For this review, take the finished solid that the model builds, in its own axes (mm). Face numbers are marked on the shaded views. A direction names the side the tool comes from. Coordinates: 2 decimals unless noted, no trailing zeros. Loops run counter-clockwise (first coordinate to the right, second up) from the corner with the lowest first, then second, coordinate; pieces in that order, holes last. Notation, with made-up numbers: M -30,0.25 L 29,0.25 A7 cw 29,13.25 Z; hole C 3.25,84 d3. An arc over 180 degrees is marked long. Answer as a JSON object with one key per item and string values. Group by question number.
Item 1: Wall thickness on L1, parallel to X at y = 32.5, z = 8.5; L2, parallel to X at y = 25.5, z = 23.5; L3, parallel to Y at x = 141.15, z = 5.75 (3 decimals): over which ranges is each line inside the solid? List them lowest first. Write a range as from..to.
Item 2: Add section A-A (y = 26.35). State the section outline as (x, z) points.
Item 3: Add section C-C (x = 49). State the section outline as (y, z) points (3 decimals).
Item 4: Tool access review of the marked faces 4, 5 and 6: name each direction out of +Z, -Z, +X, -X, +Y, -Y from which nothing blocks a thin tool from reaching the whole face with its end or side.
Item 5: Mouldability with a two-part tool opening along X and no side actions: class the marked faces 1, 2 and 3 as +X half, -X half, draft (parallel to the pull), parting line (faces both ways), or undercut.
Item 6: Insertion check: pin 1 (4 mm diameter, centred on x = 108.5, y = 29.5, fed in from +Z); pin 2 (6.5 mm diameter, centred on x = 61.5, y = 3.5, fed in from -Z); pin 3 (1.7 mm diameter, centred on x = 67.5, y = 1.5, fed in from +Z). Each pin has a flat end and moves straight along its axis. Give the tip position at first contact, or say it passes through.
Item 7: Add section D-D (x = 13.85). Count the separate pieces of the cut face and the enclosed holes in it, then the cut area to 3 significant figures.
Item 8: Add section B-B (z = -14). State the section outline as (x, y) points.
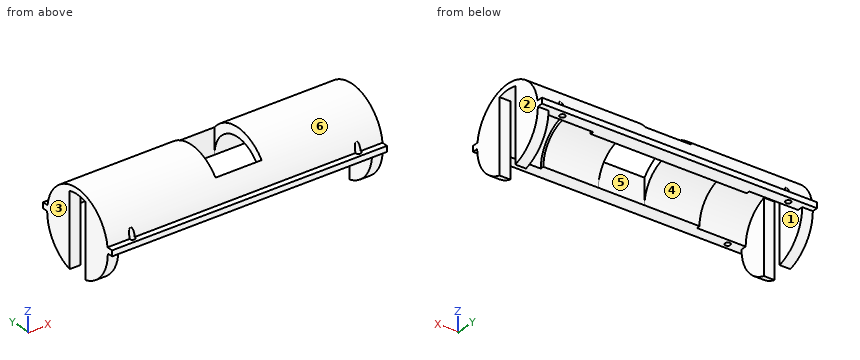
from build123d import *

# Parameters (mm, degrees)
BOSS_EXTRUDE1_DEPTH     = 155
CUT_EXTRUDE1_DEPTH      = 33.5
CUT_EXTRUDE2_START      = -33.5
CUT_EXTRUDE2_DEPTH      = 33.5
CUT_EXTRUDE3_DEPTH      = 166.346214426
CUT_EXTRUDE3_DEPTH_BACK = 166.346214426
SKETCH4_W               = 26
SKETCH4_H               = 36
CUT_EXTRUDE4_DEPTH      = 166.346214426
CUT_EXTRUDE4_DEPTH_BACK = 166.346214426
SKETCH5_R               = 1.5
BOSS_EXTRUDE2_START     = -6
BOSS_EXTRUDE2_DEPTH     = 6


with BuildPart() as part:
    # Sketch1 → Boss-Extrude1 (new body)
    with BuildSketch(Plane(origin=(0, 0, 0), x_dir=(0, 0, -1), z_dir=(1, 0, 0))):
        with BuildLine():
            Line((-6.678129735, 49.283191466), (-6.514064867, 52.7))
            Line((-6.514064867, 52.7), (-3.339064867, 52.7))
            Line((-3.339064867, 52.7), (-3.339064867, 44.35))
            ThreePointArc((-3.339064867, 44.35), (-21.339064867, 26.35), (-3.339064867, 8.35))
            Line((-3.339064867, 8.35), (-3.339064867, 0))
            Line((-3.339064867, 0), (-6.514064867, 0))
            Line((-6.514064867, 0), (-6.514064867, 3.393519434))
            ThreePointArc((-6.514064867, 3.393519434), (-26.513916757, 26.267145213), (-6.678129735, 49.283191466))
        make_face()
    extrude(amount=BOSS_EXTRUDE1_DEPTH)

    # Sketch2 → Cut-Extrude1 (cut)
    with BuildSketch(Plane(origin=(155, 0, 0), x_dir=(0, 0, -1), z_dir=(1, 0, 0))):
        with BuildLine():
            Line((-3.339064867, 46.35), (-3.339064867, 6.35))
            ThreePointArc((-3.339064867, 6.35), (-23.339064867, 26.35), (-3.339064867, 46.35))
        make_face()
    extrude(amount=-CUT_EXTRUDE1_DEPTH, mode=Mode.SUBTRACT)

    # Sketch3 → Cut-Extrude2 (cut)
    with BuildSketch(Plane.ZY.offset(CUT_EXTRUDE2_START)):
        with BuildLine():
            Line((3.339064867, 46.35), (3.339064867, 6.35))
            ThreePointArc((3.339064867, 6.35), (23.339064867, 26.35), (3.339064867, 46.35))
        make_face()
    extrude(amount=CUT_EXTRUDE2_DEPTH, mode=Mode.SUBTRACT)

    # Sketch4 → Cut-Extrude3 (cut, two sides: drawn at the far end of the back side and taken through both)
    with BuildSketch(Plane(origin=(0, 0, 3.339064867), x_dir=(-1, 0, 0), z_dir=(0, 0, -1)).offset(-CUT_EXTRUDE3_DEPTH_BACK)):
        with Locations((-77.5, 26.35)):
            Rectangle(SKETCH4_W, SKETCH4_H)
    extrude(amount=CUT_EXTRUDE3_DEPTH + CUT_EXTRUDE3_DEPTH_BACK, mode=Mode.SUBTRACT)

    # Sketch5 → Cut-Extrude4 (cut, two sides: drawn at the far end of the back side and taken through both)
    with BuildSketch(Plane(origin=(0, 0, 3.339064867), x_dir=(-1, 0, 0), z_dir=(0, 0, -1)).offset(-CUT_EXTRUDE4_DEPTH_BACK)):
        with Locations(Location((-141.15, 49.525, 0), (0, 0, 350.723114584))):
            Circle(SKETCH5_R)
        with Locations(Location((-141.15, 3.175, 0), (0, 0, 8.376636586))):
            Circle(SKETCH5_R)
        with Locations(Location((-13.85, 49.525, 0), (0, 0, 350.723114584))):
            Circle(SKETCH5_R)
        with Locations(Location((-13.85, 3.175, 0), (0, 0, 8.376636586))):
            Circle(SKETCH5_R)
    extrude(amount=CUT_EXTRUDE4_DEPTH + CUT_EXTRUDE4_DEPTH_BACK, mode=Mode.SUBTRACT)

    # Sketch6 → Boss-Extrude2 (add)
    with BuildSketch(Plane(origin=(155, 0, 0), x_dir=(0, 0, -1), z_dir=(1, 0, 0)).offset(BOSS_EXTRUDE2_START)):
        with BuildLine():
            Line((-25.72389511, 32.35), (19.045765375, 32.35))
            ThreePointArc((19.045765375, 32.35), (-3.339064867, 49.525), (-25.72389511, 32.35))
        make_face()
        with BuildLine():
            Line((-25.72389511, 20.35), (19.045765375, 20.35))
            ThreePointArc((19.045765375, 20.35), (-3.339064867, 3.175), (-25.72389511, 20.35))
        make_face()
    boss_extrude2 = extrude(amount=BOSS_EXTRUDE2_DEPTH)

    # Mirror1: Boss-Extrude2 across plane
    add(boss_extrude2.mirror(Plane(origin=(77.5, 0, 0), x_dir=(0, 0, 1), z_dir=(1, 0, 0))))


solid = part.part
From the geometry:
{
 "1": {"L1": "x = 0..6, 149..155", "L2": "x = 0..64.5, 90.5..155", "L3": "y = 0..1.675, 4.675..6.496, 46.204..48.025, 51.025..52.7"},
 "2": {"outline": "M 0,23.34 L 33.5,23.34 L 33.5,21.34 L 64.5,21.34 L 64.5,26.51 L 0,26.51 Z; M 90.5,21.34 L 121.5,21.34 L 121.5,23.34 L 155,23.34 L 155,26.51 L 90.5,26.51 Z"},
 "3": {"outline": "M 0,3.339 L 8.35,3.339 A18 cw 44.35,3.339 L 52.7,3.339 L 52.7,6.514 L 49.283,6.678 A23.175 ccw 3.394,6.514 L 0,6.514 Z"},
 "4": {"face 4": "-Z", "face 5": "+Z, -Z", "face 6": "+Z, +X, -X"},
 "5": {"face 1": "undercut", "face 2": "+X half", "face 3": "-X half"},
 "6": {"pin 1": "stops at z = 26.49", "pin 2": "stops at z = 3.34", "pin 3": "stops at z = 6.51"},
 "7": {"separate pieces": "3", "enclosed holes": "0", "area": "210 mm²"},
 "8": {"outline": "M 0,10.97 L 6,10.97 L 6,20.35 L 0,20.35 Z; M 0,32.35 L 6,32.35 L 6,41.73 L 0,41.73 Z; M 149,10.97 L 155,10.97 L 155,20.35 L 149,20.35 Z; M 149,32.35 L 155,32.35 L 155,41.73 L 149,41.73 Z"}
}
